```python
from build123d import *

# Parameters (mm, degrees)
SKETCH_1_W          = 58
SKETCH_1_H          = 58
SKETCH_1_R          = 2
EXTRUDE_1_DEPTH     = 3
FILLET_2_R          = 5
FILLET_3_R          = 5
FILLET_4_R          = 5
FILLET_5_R          = 5
SKETCH_2_R          = 3
CUT_EXTRUDE_1_DEPTH = 3


with BuildPart() as part:
    # Эскиз1 → Бобышка-Вытянуть1 (new body)
    with BuildSketch(Plane.XY):
        Rectangle(SKETCH_1_W, SKETCH_1_H)
        with Locations((0, 25)):
            Circle(SKETCH_1_R, mode=Mode.SUBTRACT)
        with Locations(Location((-25, 0, 0), (0, 0, 180))):
            Circle(SKETCH_1_R, mode=Mode.SUBTRACT)
        with Locations(Location((0, -25, 0), (0, 0, 180))):
            Circle(SKETCH_1_R, mode=Mode.SUBTRACT)
        with Locations(Location((25, 0, 0), (0, 0, 180))):
            Circle(SKETCH_1_R, mode=Mode.SUBTRACT)
    extrude(amount=EXTRUDE_1_DEPTH)

    # Скругление2
    fillet_2_edges = [part.edges().sort_by_distance(p)[0] for p in [
        (29, -29, 1.5),
    ]]
    fillet(fillet_2_edges, radius=FILLET_2_R)

    # Скругление3
    fillet_3_edges = [part.edges().sort_by_distance(p)[0] for p in [
        (-29, -29, 1.5),
    ]]
    fillet(fillet_3_edges, radius=FILLET_3_R)

    # Скругление4
    fillet_4_edges = [part.edges().sort_by_distance(p)[0] for p in [
        (-29, 29, 1.5),
    ]]
    fillet(fillet_4_edges, radius=FILLET_4_R)

    # Скругление5
    fillet_5_edges = [part.edges().sort_by_distance(p)[0] for p in [
        (29, 29, 1.5),
    ]]
    fillet(fillet_5_edges, radius=FILLET_5_R)

    # Эскиз2 → Вырез-Вытянуть1 (cut)
    with BuildSketch(Plane.XY.offset(3)):
        Circle(SKETCH_2_R)
    extrude(amount=-CUT_EXTRUDE_1_DEPTH, mode=Mode.SUBTRACT)


solid = part.part
```
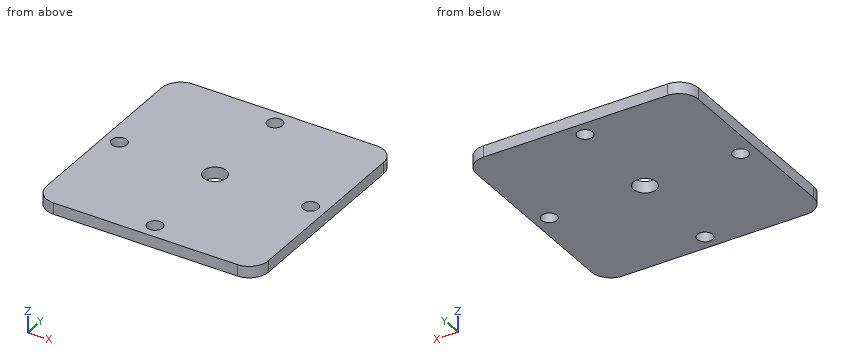
The listing builds one solid part. Answer for the finished solid, in the listing's coordinates (mm). Give positions to 0.01 mm unless a question says otherwise; leave off trailing zeros. Loops run counter-clockwise (first coordinate to the right, second up) from the corner with the lowest first, then second, coordinate; pieces in that order, holes last. Notation, with made-up numbers: (72, 23) - (83, 23) arc R12 cw to (83, 42) - close; hole circle Ø8 at (-3.5, -36.5). An arc over 180 degrees is marked (long way). Answer as CSV lines item,"result". Start each with the question number.
Item 1: A cutting plane is placed at B-B on y = 0. Determine the outline of the cut face in (x, z).
Item 2: A cutting plane is placed at A-A on z = 1.7. Determine the outline of the cut face in (x, y), then the cut area to 3 significant figures.
Item 3: This flat-tipped pin is pushed along its axis until it touches: pin 1 (3.5 mm diameter, centred on x = 0, y = 25, fed in from +Z). Where does it stop, or does it pass through?
Item 4: A cutting plane is placed at C-C on x = 25. Determine the outline of the cut face in (y, z), then the cut area to 3 significant figures.
Item 5: Find the intervals of material crossed by line 1 (Y direction, x = 0, z = 2.15); line 2 (Y direction, x = -0.5, z = 0.2); line 3 (X direction, y = 26, z = 1.7), in increasing order. Write a range as from..to.
Item 6: A cutting plane is placed at D-D on x = 1. Determine the outline of the cut face in (y, z), then the cut area to 3 significant figures.
Found:
1,outline,"(-29, 0) - (-27, 0) - (-27, 3) - (-29, 3) - close; (-23, 0) - (-3, 0) - (-3, 3) - (-23, 3) - close; (3, 0) - (23, 0) - (23, 3) - (3, 3) - close; (27, 0) - (29, 0) - (29, 3) - (27, 3) - close"
2,outline,"(-29, -24) arc R5 ccw to (-24, -29) - (24, -29) arc R5 ccw to (29, -24) - (29, 24) arc R5 ccw to (24, 29) - (-24, 29) arc R5 ccw to (-29, 24) - close; hole circle Ø4 at (-25, 0); hole circle Ø6 at (0, 0); hole circle Ø4 at (0, -25); hole circle Ø4 at (0, 25); hole circle Ø4 at (25, 0)"
2,area,"3,260 mm^2"
3,pin 1,"passes through"
4,outline,"(-28.9, 0) - (-2, 0) - (-2, 3) - (-28.9, 3) - close; (2, 0) - (28.9, 0) - (28.9, 3) - (2, 3) - close"
4,area,"161 mm^2"
5,line 1,"y = -29..-27, -23..-3, 3..23, 27..29"
5,line 2,"y = -29..-26.94, -23.06..-2.96, 2.96..23.06, 26.94..29"
5,line 3,"x = -28.58..-1.73, 1.73..28.58"
6,outline,"(-29, 0) - (-26.73, 0) - (-26.73, 3) - (-29, 3) - close; (-23.27, 0) - (-2.83, 0) - (-2.83, 3) - (-23.27, 3) - close; (2.83, 0) - (23.27, 0) - (23.27, 3) - (2.83, 3) - close; (26.73, 0) - (29, 0) - (29, 3) - (26.73, 3) - close"
6,area,"136 mm^2"
